Could you check a few things on this model? Use its own coordinates, in mm. A direction names the side the tool comes from. Give positions to 0.01 mm unless a question says otherwise; leave off trailing zeros. Answer as CSV lines item,"result". Start each with the question number.
from build123d import *

# Parameters (mm, degrees)
EXTRUDE_THIN1_DEPTH = 508
FILLET1_R           = 1.016


with BuildPart() as part:
    # Sketch1 → Extrude-Thin1 (new body)
    with BuildSketch(Plane.XY):
        with BuildLine():
            Line((0, 3.175), (0, 0))
            Line((0, 0), (-7.9375, 0))
            Line((-7.9375, 0), (-7.9375, 9.525))
            ThreePointArc((-7.9375, 9.525), (-10.26234, 15.13766), (-15.875, 17.4625))
            Line((-15.875, 17.4625), (-15.875, 23.8125))
            ThreePointArc((-15.875, 23.8125), (-23.732724, 27.067276), (-26.9875, 34.925))
            Line((-26.9875, 34.925), (-28.575, 34.925))
            Line((-28.575, 34.925), (-28.575, 47.625))
            Line((-28.575, 47.625), (0, 47.625))
            Line((0, 47.625), (0, 44.45))
            Line((0, 44.45), (-1.016, 44.45))
            Line((-1.016, 44.45), (-1.016, 46.609))
            Line((-1.016, 46.609), (-27.559, 46.609))
            Line((-27.559, 46.609), (-27.559, 35.941))
            Line((-27.559, 35.941), (-25.92025, 35.941))
            ThreePointArc((-25.92025, 35.941), (-23.014304, 27.785696), (-14.859, 24.87975))
            Line((-14.859, 24.87975), (-14.859, 18.420668))
            ThreePointArc((-14.859, 18.420668), (-9.194359, 15.486057), (-6.9215, 9.525))
            Line((-6.9215, 9.525), (-6.9215, 1.016))
            Line((-6.9215, 1.016), (-1.016, 1.016))
            Line((-1.016, 1.016), (-1.016, 3.175))
            Line((-1.016, 3.175), (0, 3.175))
        make_face()
    extrude(amount=-EXTRUDE_THIN1_DEPTH)

    # Fillet1
    fillet1_edges = [part.edges().sort_by_distance(p)[0] for p in [
        (-25.92025, 35.941, -254),
        (-14.859, 24.87975, -254),
        (0, 0, -254),
        (-7.9375, 0, -254),
        (-15.875, 17.4625, -254),
        (-28.575, 34.925, -254),
        (-28.575, 47.625, -254),
        (0, 47.625, -254),
    ]]
    fillet(fillet1_edges, radius=FILLET1_R)


solid = part.part
1. Will these pins go through, and if not, where does the flat tip stop? P1, Ø1.5, axis at x = -15.5, z = -55.5, coming from the -Y side; P2, Ø2.5, axis at y = 21.5, z = -180, coming from the +X side; P3, Ø0.8, axis at x = -0.5, z = -262.5, coming from the +Y side.
2. Please list where these lines run through material, in increasing order: line 1 (Y direction, x = -5, z = -108) (3 decimals); line 2 (Y direction, x = -14.5, z = -204) (1 decimal); line 3 (X direction, y = 45.5, z = -397) (3 decimals).
3. Thinking about a two-plate mould opening in X: for faces 1 (the flat face through (-6.922, 5, -250)), 2 (the flat face through (-15.3, 23.9, 0)), 3 (the flat face through (-7.938, 5, -250)), which applies, pulls with the +X half, pulls with the -X half, needs draft (parallel to the pull), parting line crosses it, or undercut?
4. On a 3-axis mill with a long thin cutter (end or side, diameter ignored), from which of +Z, -Z, +X, -X, +Y, -Y can I reach the whole of each face in a straight line? I mean faces 4 (the flat face through (-15.3, 23.9, -508)), 5 (the cylindrical face through (-9.3, 15.6, -250.4)), 6 (the flat face through (-14, 46.609, -250)). Say none if no direction works.
Solutions:
1,P1,"y = 17.38"
1,P2,"x = -14.86"
1,P3,"y = 47.62"
2,line 1,"0 to 1.016, 46.609 to 47.625"
2,line 2,"17.3 to 18.4, 46.6 to 47.6"
2,line 3,"-28.575 to -27.559, -1.016 to 0"
3,face 1,"undercut"
3,face 2,"needs draft"
3,face 3,"pulls with the -X half"
4,face 4,"-Z, +X, -X, +Y, -Y"
4,face 5,"+Z, -Z, +X"
4,face 6,"+Z, -Z"
